from build123d import *

# Parameters (mm, degrees)
SCHIZZO1_R               = 12.5
ESTRUSIONE1_DEPTH        = 510
SCHIZZO2_R               = 4
TAGLIO_ESTRUSIONE1_DEPTH = 30
TAGLIO_ESTRUSIONE2_START = -30
SCHIZZO3_R               = 4
TAGLIO_ESTRUSIONE2_DEPTH = 30
SCHIZZO5_W               = 1.3
SCHIZZO5_H               = 0.55


with BuildPart() as part:
    # Schizzo1 → Estrusione1 (new body)
    with BuildSketch(Plane.XY):
        Circle(SCHIZZO1_R)
    extrude(amount=ESTRUSIONE1_DEPTH)

    # Schizzo2 → Taglio-Estrusione1 (cut)
    with BuildSketch(Plane.XY.offset(510)):
        Circle(SCHIZZO2_R)
    extrude(amount=-TAGLIO_ESTRUSIONE1_DEPTH, mode=Mode.SUBTRACT)

    # Schizzo3 → Taglio-Estrusione2 (cut)
    with BuildSketch(Plane(origin=(0, 0, 0), x_dir=(-1, 0, 0), z_dir=(0, 0, -1)).offset(TAGLIO_ESTRUSIONE2_START)):
        with Locations(Location((0, 0, 0), (0, 0, 180))):
            Circle(SCHIZZO3_R)
    extrude(amount=TAGLIO_ESTRUSIONE2_DEPTH, mode=Mode.SUBTRACT)

    # Schizzo5 → Taglia-Rivoluzione1 (revolve, cut)
    with BuildSketch(Plane(origin=(0, 0, 0), x_dir=(0, 0, -1), z_dir=(1, 0, 0)), mode=Mode.PRIVATE) as taglia_rivoluzione1_sk:
        with Locations((-508.35, 12.225)):
            Rectangle(SCHIZZO5_W, SCHIZZO5_H)
        with Locations((-1.65, 12.225)):
            Rectangle(SCHIZZO5_W, SCHIZZO5_H)
    revolve(taglia_rivoluzione1_sk.sketch.rotate(Axis((0, 0, 510), (0, 0, -1)), 90), axis=Axis((0, 0, 510), (0, 0, -1)), mode=Mode.SUBTRACT)


solid = part.part
Model file for the job. Use its own axes, mm. A direction names the side the tool comes from. Give positions to 0.01 mm unless a question says otherwise; leave off trailing zeros. Loops run counter-clockwise (first coordinate to the right, second up) from the corner with the lowest first, then second, coordinate; pieces in that order, holes last.
1) Pull direction Z, two halves, no side cores. Call faces 1 (the cylindrical face through (-0.867, 3.905, 15.21)), 2 (the cylindrical face through (6.42, -10.08, 1.64)), 3 (the flat face through (0, 0, 30)): +Z half, -Z half, draft (parallel to the pull), parting line (faces both ways), or undercut.
2) Wall check: line 1 (Y direction, x = 0, z = 20.25); line 2 (X direction, y = -3.5, z = 124); line 3 (X direction, y = 3.75, z = 132.5). Give the ranges that are in metal, low to high.
3) Tool access for faces 4 (the flat face through (-3, 3, 510)), 5 (the cylindrical face through (-0.867, -3.905, 495.21)), 6 (the cylindrical face through (6.42, -10.08, 508.34)): list every direction of +Z, -Z, +X, -X, +Y, -Y with a clear straight run to the whole face (end or side of a thin tool).
4) Saw through at A-A (y = 0). Write the cut outline in (x, z).
5) Saw through at C-C (z = 442). Write the cut outline in (x, y), plus the area to 3 significant figures.
6) Flat gauge pin, fed straight in: pin 1 Ø7 at (x, y) = (0, 0) entering from -Z. Where does the tip first touch, or does it go through?
Answer block:
1. face 1: draft
1. face 2: undercut
1. face 3: -Z half
2. line 1: y = -12.5 to -4, 4 to 12.5
2. line 2: x = -12 to 12
2. line 3: x = -11.92 to 11.92
3. face 4: +Z, +X, -X, +Y, -Y
3. face 5: +Z
3. face 6: none
4. outline: (-12.5, 0) - (-4, 0) - (-4, 30) - (4, 30) - (4, 0) - (12.5, 0) - (12.5, 1) - (11.95, 1) - (11.95, 2.3) - (12.5, 2.3) - (12.5, 507.7) - (11.95, 507.7) - (11.95, 509) - (12.5, 509) - (12.5, 510) - (4, 510) - (4, 480) - (-4, 480) - (-4, 510) - (-12.5, 510) - (-12.5, 509) - (-11.95, 509) - (-11.95, 507.7) - (-12.5, 507.7) - (-12.5, 2.3) - (-11.95, 2.3) - (-11.95, 1) - (-12.5, 1) - close
5. outline: circle Ø25 at (0, 0)
5. area: 491 mm2
6. pin 1: stops at z = 30
